from build123d import *

# Parameters (mm, degrees)
SKETCH001_W             = 300
SKETCH001_H             = 350
PAD001_DEPTH            = 1.6
PAD002_DEPTH            = 1.6
BODY001_PLACEMENT_ANGLE = 180


with BuildPart() as part:
    # Sketch001 → Pad001 (new body)
    with BuildSketch(Plane.XY):
        Rectangle(SKETCH001_W, SKETCH001_H)
    extrude(amount=PAD001_DEPTH)

    with BuildSketch(Plane(origin=(-150, 0, 0), x_dir=(0.717792, 0, -0.696258), z_dir=(0.696258, 0, 0.717792))):
        Polygon((0, -175), (0, 175), (-139.316187, 6), (-139.316187, -6), align=None)
    pad002 = extrude(amount=PAD002_DEPTH)

    # Mirrored: Pad002 across YZ
    add(pad002.mirror(Plane.YZ))


with BuildPart() as part_1:
    # Body001 placement: moved
    add(part.part.moved(Location((0, 0, 100))).rotate(Axis((0, 0, 100), (1, 0, 0)), BODY001_PLACEMENT_ANGLE))


solid = part_1.part
Input: part model. Units: mm. Frame: model coordinates. A direction names the side the tool comes from. Coordinates: 2 decimals unless noted, no trailing zeros. Loops run counter-clockwise (first coordinate to the right, second up) from the corner with the lowest first, then second, coordinate; pieces in that order, holes last.
Q1. Contact query for flat-ended pins moving along their axis: pin 1 (0.7 mm diameter, centred on y = -174.5, z = 99, fed in from -X); pin 2 (1.1 mm diameter, centred on y = -174, z = 99.5, fed in from +X); pin 3 (4 mm diameter, centred on y = -21, z = 47.5, fed in from -X); pin 4 (10 mm diameter, centred on y = -97.5, z = 45.5, fed in from -X). Output: stop coordinate, or through.
Q2. Cut plane B-B (y = -127.5). Output: boundary loops of the cut face in (x, z).
Q3. Draft query along X for faces 1 (the face through (-2, -2, 100)), 2 (the face through (188.756, -2.439, 60.178)), 3 (the face through (198.75, -91.68, 51.61)). Return one class per face: +X half, -X half, draft (parallel to the pull), parting line (faces both ways), or undercut.
Q4. Set-up query: faces 4 (the face through (-2, -2, 98.4)), 5 (the face through (-189.59, -2.45, 61.6)). Return all of +Z, -Z, +X, -X, +Y, -Y with unobstructed straight access to the full face (end or side cutting, diameter ignored); none if empty.
Q5. Material intervals for line 1 (Z direction, x = 76, y = 41.5); line 2 (X direction, y = 72, z = 52); line 3 (X direction, y = 12, z = 90.5), sorted ascending.
Q6. Cut plane A-A (z = 48). Output: boundary loops of the cut face in (x, y).
Q7. Cut plane C-C (x = 58). Output: boundary loops of the cut face in (y, z).
Q8. Cut plane D-D (z = 82.5). Output: boundary loops of the cut face in (x, y).
Working result:
1. pin 1: stops at x = -150.13
1. pin 2: stops at x = 150.85
1. pin 3: stops at x = -206.19
1. pin 4: passes through
2. outline: (-178.11, 72.74) - (-176.99, 71.59) - (-149.35, 98.4) - (149.35, 98.4) - (176.99, 71.59) - (178.11, 72.74) - (150, 100) - (-150, 100) - close
3. face 1: draft
3. face 2: undercut
3. face 3: +X half
4. face 4: -Z, +Y, -Y
4. face 5: +Z, -X, +Y, -Y
5. line 1: z = 98.4 to 100
5. line 2: x = -199.48 to -197.19, 197.19 to 199.48
5. line 3: x = -159.79 to -157.5, 157.5 to 159.79
6. outline: (-203.61, -84.4) - (-201.31, -86.4) - (-201.31, 86.4) - (-203.61, 84.4) - close; (201.31, -86.4) - (203.61, -84.4) - (203.61, 84.4) - (201.31, 86.4) - close
7. outline: (-175, 98.4) - (175, 98.4) - (175, 100) - (-175, 100) - close
8. outline: (-168.04, -144.51) - (-165.74, -146.51) - (-165.74, 146.51) - (-168.04, 144.51) - close; (165.74, -146.51) - (168.04, -144.51) - (168.04, 144.51) - (165.74, 146.51) - close
